Work out the finished part from the listing and answer in its coordinate system (mm). A direction names the side the tool comes from. Coordinates: 2 decimals unless noted, no trailing zeros. Order: outer loops, then holes, each group sorted by start corner. A loop starts at its lowest first (then second) coordinate and runs counter-clockwise, first axis right, second up. Notation, with made-up numbers: M 11.5,-38.75 L 64.5,-38.75 A29 ccw 64.5,-11.75 Z; hole C 32.25,46.25 d2. An arc over 180 degrees is marked long. Use a Markdown table: item, result.
from build123d import *

# Parameters (mm, degrees)
SKETCH1_R                       = 1.15
BOSS_EXTRUDE4_DEPTH             = 3.22
BOSS_EXTRUDE5_DEPTH             = 19
BOSS_EXTRUDE6_DEPTH             = 19
SKETCH3_W                       = 19
SKETCH3_H                       = 8.72
CUT_EXTRUDE1_DEPTH              = 93.159937036
SKETCH2_5_R                     = 6.5
SKETCH2_5_R_2                   = 2.25
SKETCH2_5_W                     = 6.12
SKETCH2_5_H                     = 9.37
BOSS_EXTRUDE9_DEPTH             = 3
BOSS_EXTRUDE9_DEPTH_BACK        = 2
CUT_EXTRUDE8_REACH              = 94.16
SKETCH2_6_W                     = 64
SKETCH2_6_H                     = 14.977988196
CUT_EXTRUDE8_DIRECTION_2_REACH  = 94.16
CUT_EXTRUDE10_REACH             = 94.825
SKETCH4_W                       = 22.69
SKETCH4_H                       = 19
CUT_EXTRUDE10_DIRECTION_2_DEPTH = 3
CUT_EXTRUDE11_REACH             = 93.768
SKETCH5_W                       = 12.894145303
SKETCH5_H                       = 8.72


with BuildPart() as part:
    # Sketch1 → Boss-Extrude4 (new body)
    with BuildSketch(Plane.XY):
        with BuildLine():
            ThreePointArc((2.480923897, -4.488118441), (3.840990258, -3.840990258), (4.488118441, -2.480923897))
            Line((4.488118441, -2.480923897), (2.480923897, -4.488118441))
        make_face()
        with BuildLine():
            Line((2.480923897, -4.488118441), (4.488118441, -2.480923897))
            ThreePointArc((4.488118441, -2.480923897), (4.497027647, -2.365614681), (4.5, -2.25))
            ThreePointArc((4.5, -2.25), (0.579359589, -0.742863438), (2.480923897, -4.488118441))
        make_face()
        with Locations(Location((2.25, -2.25, 0), (0, 0, 180))):
            Circle(SKETCH1_R, mode=Mode.SUBTRACT)
        with BuildLine():
            ThreePointArc((4.5, -47.75), (4.497027647, -47.634385319), (4.488118441, -47.519076103))
            Line((4.488118441, -47.519076103), (2.480923897, -45.511881559))
            ThreePointArc((2.480923897, -45.511881559), (0.579359589, -49.257136562), (4.5, -47.75))
        make_face()
        with Locations(Location((2.25, -47.75, 0), (0, 0, 180))):
            Circle(SKETCH1_R, mode=Mode.SUBTRACT)
        with BuildLine():
            Line((2.480923897, -45.511881559), (4.488118441, -47.519076103))
            ThreePointArc((4.488118441, -47.519076103), (3.840990258, -46.159009742), (2.480923897, -45.511881559))
        make_face()
        with BuildLine():
            Line((67.519076103, -45.511881559), (65.511881559, -47.519076103))
            ThreePointArc((65.511881559, -47.519076103), (67.634385319, -49.997027647), (70, -47.75))
            ThreePointArc((70, -47.75), (69.257136562, -46.079359589), (67.519076103, -45.511881559))
        make_face()
        with Locations(Location((67.75, -47.75, 0), (0, 0, 180))):
            Circle(SKETCH1_R, mode=Mode.SUBTRACT)
        with BuildLine():
            ThreePointArc((67.519076103, -45.511881559), (66.159009742, -46.159009742), (65.511881559, -47.519076103))
            Line((65.511881559, -47.519076103), (67.519076103, -45.511881559))
        make_face()
        with BuildLine():
            ThreePointArc((70, -2.25), (67.634385319, -0.002972353), (65.511881559, -2.480923897))
            Line((65.511881559, -2.480923897), (67.519076103, -4.488118441))
            ThreePointArc((67.519076103, -4.488118441), (69.257136562, -3.920640411), (70, -2.25))
        make_face()
        with Locations(Location((67.75, -2.25, 0), (0, 0, 180))):
            Circle(SKETCH1_R, mode=Mode.SUBTRACT)
        with BuildLine():
            Line((67.519076103, -4.488118441), (65.511881559, -2.480923897))
            ThreePointArc((65.511881559, -2.480923897), (66.159009742, -3.840990258), (67.519076103, -4.488118441))
        make_face()
    extrude(amount=BOSS_EXTRUDE4_DEPTH)

    # Sketch1<6> → Boss-Extrude5 (add)
    with BuildSketch(Plane.XY):
        with BuildLine():
            Line((65.511881559, -47.519076103), (63.030957663, -50))
            ThreePointArc((63.030957663, -50), (71.446745906, -51.446745906), (70, -43.030957663))
            Line((70, -43.030957663), (67.519076103, -45.511881559))
            ThreePointArc((67.519076103, -45.511881559), (69.340990258, -49.340990258), (65.511881559, -47.519076103))
        make_face()
        with BuildLine():
            ThreePointArc((70, -6.969042337), (71.446745906, 1.446745906), (63.030957663, 0))
            Line((63.030957663, 0), (65.511881559, -2.480923897))
            ThreePointArc((65.511881559, -2.480923897), (69.340990258, -0.659009742), (67.519076103, -4.488118441))
            Line((67.519076103, -4.488118441), (70, -6.969042337))
        make_face()
        with BuildLine():
            Line((4.488118441, -2.480923897), (6.969042337, 0))
            ThreePointArc((6.969042337, 0), (-1.446745906, 1.446745906), (0, -6.969042337))
            Line((0, -6.969042337), (2.480923897, -4.488118441))
            ThreePointArc((2.480923897, -4.488118441), (0.659009742, -0.659009742), (4.488118441, -2.480923897))
        make_face()
        with BuildLine():
            ThreePointArc((0, -43.030957663), (-1.446745906, -51.446745906), (6.969042337, -50))
            Line((6.969042337, -50), (4.488118441, -47.519076103))
            ThreePointArc((4.488118441, -47.519076103), (0.659009742, -49.340990258), (2.480923897, -45.511881559))
            Line((2.480923897, -45.511881559), (0, -43.030957663))
        make_face()
    extrude(amount=BOSS_EXTRUDE5_DEPTH)

    # Sketch2 → Boss-Extrude6 (add)
    with BuildSketch(Plane.XY.offset(19)):
        with BuildLine():
            Line((0, -43.030957663), (0, -6.969042337))
            ThreePointArc((0, -6.969042337), (-2.171246093, -5.040061571), (-2.977988196, -2.25))
            Line((-2.977988196, -2.25), (-2.977988196, -47.75))
            ThreePointArc((-2.977988196, -47.75), (-2.171246093, -44.959938429), (0, -43.030957663))
        make_face()
        with BuildLine():
            Line((67.75, 2.977988196), (2.25, 2.977988196))
            ThreePointArc((2.25, 2.977988196), (5.040061571, 2.171246093), (6.969042337, 0))
            Line((6.969042337, 0), (63.030957663, 0))
            ThreePointArc((63.030957663, 0), (64.959938429, 2.171246093), (67.75, 2.977988196))
        make_face()
        with BuildLine():
            Line((2.25, -52.977988196), (67.75, -52.977988196))
            ThreePointArc((67.75, -52.977988196), (64.959938429, -52.171246093), (63.030957663, -50))
            Line((63.030957663, -50), (6.969042337, -50))
            ThreePointArc((6.969042337, -50), (5.040061571, -52.171246093), (2.25, -52.977988196))
        make_face()
        with BuildLine():
            Line((72.977988196, -47.75), (72.977988196, -2.25))
            ThreePointArc((72.977988196, -2.25), (72.171246093, -5.040061571), (70, -6.969042337))
            Line((70, -6.969042337), (70, -43.030957663))
            ThreePointArc((70, -43.030957663), (72.171246093, -44.959938429), (72.977988196, -47.75))
        make_face()
    extrude(amount=-BOSS_EXTRUDE6_DEPTH)

    # Sketch3 → Cut-Extrude1 (cut, through all)
    with BuildSketch(Plane(origin=(0, 0, 0), x_dir=(0, 0, -1), z_dir=(1, 0, 0))):
        with Locations((-9.5, -13.08)):
            Rectangle(SKETCH3_W, SKETCH3_H)
    extrude(amount=-CUT_EXTRUDE1_DEPTH, mode=Mode.SUBTRACT)

    # Sketch2<5> → Boss-Extrude9 (add, two sides)
    with BuildSketch(Plane.XY.offset(19)) as boss_extrude9_sk:
        with BuildLine():
            Line((2.25, -52.977988196), (67.75, -52.977988196))
            ThreePointArc((67.75, -52.977988196), (71.446745906, -51.446745906), (72.977988196, -47.75))
            Line((72.977988196, -47.75), (72.977988196, -2.25))
            ThreePointArc((72.977988196, -2.25), (71.446745906, 1.446745906), (67.75, 2.977988196))
            Line((67.75, 2.977988196), (2.25, 2.977988196))
            ThreePointArc((2.25, 2.977988196), (-1.446745906, 1.446745906), (-2.977988196, -2.25))
            Line((-2.977988196, -2.25), (-2.977988196, -47.75))
            ThreePointArc((-2.977988196, -47.75), (-1.446745906, -51.446745906), (2.25, -52.977988196))
        make_face()
        with BuildLine():
            Line((3, -50), (2.25, -50))
            ThreePointArc((2.25, -50), (0.032403241, -47.369520548), (3, -45.628679656))
            Line((3, -45.628679656), (3, -50))
        make_face(mode=Mode.SUBTRACT)
        with Locations((17.28, -30.89)):
            Circle(SKETCH2_5_R, mode=Mode.SUBTRACT)
        with BuildLine():
            ThreePointArc((67, -45.628679656), (69.967596759, -47.369520548), (67.75, -50))
            Line((67.75, -50), (67, -50))
            Line((67, -50), (67, -45.628679656))
        make_face(mode=Mode.SUBTRACT)
        with Locations(Location((2.25, -2.25, 0), (0, 0, 275.890801568))):
            Circle(SKETCH2_5_R_2, mode=Mode.SUBTRACT)
        with Locations((43.23, -13)):
            Rectangle(SKETCH2_5_W, SKETCH2_5_H, mode=Mode.SUBTRACT)
        with Locations(Location((67.75, -2.25, 0), (0, 0, 185.890801568))):
            Circle(SKETCH2_5_R_2, mode=Mode.SUBTRACT)
    extrude(amount=BOSS_EXTRUDE9_DEPTH)
    extrude(boss_extrude9_sk.sketch, amount=-BOSS_EXTRUDE9_DEPTH_BACK)

    # Sketch2<6> → Cut-Extrude8 (cut, up to next)
    with BuildSketch(Plane.XY.offset(19), mode=Mode.PRIVATE) as cut_extrude8_sk1:
        with Locations((35, -45.488994098)):
            Rectangle(SKETCH2_6_W, SKETCH2_6_H)
    cut_extrude8_tool1 = extrude(cut_extrude8_sk1.sketch, amount=-CUT_EXTRUDE8_REACH, mode=Mode.PRIVATE) & part.part
    add(cut_extrude8_tool1.solids().sort_by_distance((35, -45.488994, 19))[0], mode=Mode.SUBTRACT)

    # Sketch2<6> → Cut-Extrude8 direction 2 (cut, up to next)
    with BuildSketch(Plane.XY.offset(19), mode=Mode.PRIVATE) as cut_extrude8_direction_2_sk1:
        with Locations((35, -45.488994098)):
            Rectangle(SKETCH2_6_W, SKETCH2_6_H)
    cut_extrude8_direction_2_tool1 = extrude(cut_extrude8_direction_2_sk1.sketch, amount=CUT_EXTRUDE8_DIRECTION_2_REACH, mode=Mode.PRIVATE) & part.part
    add(cut_extrude8_direction_2_tool1.solids().sort_by_distance((35, -45.488994, 19))[0], mode=Mode.SUBTRACT)

    # Sketch4 → Cut-Extrude10 (cut, up to next)
    with BuildSketch(Plane.XZ, mode=Mode.PRIVATE) as cut_extrude10_sk1:
        with Locations((54.295, 9.5)):
            Rectangle(SKETCH4_W, SKETCH4_H)
    cut_extrude10_tool1 = extrude(cut_extrude10_sk1.sketch, amount=-CUT_EXTRUDE10_REACH, mode=Mode.PRIVATE) & part.part
    add(cut_extrude10_tool1.solids().sort_by_distance((54.295, 0, 9.5))[0], mode=Mode.SUBTRACT)

    # Sketch4 → Cut-Extrude10 direction 2 (cut)
    with BuildSketch(Plane.XZ):
        with Locations((54.295, 9.5)):
            Rectangle(SKETCH4_W, SKETCH4_H)
    extrude(amount=CUT_EXTRUDE10_DIRECTION_2_DEPTH, mode=Mode.SUBTRACT)

    # Sketch5 → Cut-Extrude11 (cut, up to next)
    with BuildSketch(Plane(origin=(0, 0, 17), x_dir=(-1, 0, 0), z_dir=(0, 0, -1)), mode=Mode.PRIVATE) as cut_extrude11_sk1:
        with Locations((-3.469084455, -13.08)):
            Rectangle(SKETCH5_W, SKETCH5_H)
    cut_extrude11_tool1 = extrude(cut_extrude11_sk1.sketch, amount=-CUT_EXTRUDE11_REACH, mode=Mode.PRIVATE) & part.part
    add(cut_extrude11_tool1.solids().sort_by_distance((3.469084, -13.08, 17))[0], mode=Mode.SUBTRACT)


solid = part.part
(1) A cutting plane is placed at B-B (x = 18). Determine the outline of the cut face in (y, z), then the cut area to 3 significant figures.
Conclusion:
| item | result |
|---|---|
| outline | M -38,17 L -37.35,17 L -37.35,22 L -38,22 Z; M -24.43,17 L 0,17 L 0,0 L 2.98,0 L 2.98,22 L -24.43,22 Z |
| area | 191 mm2 |
(2) Determine the mould class of faces 1 (the flat face through (9.916, -13, 19)), 2 (the cylindrical face through (20.279, -36.657, 19.465)), 3 (the flat face through (3, -42, 19)), 4 (the flat face through (72.978, -25, 11)) for opening direction X: pulls with the +X half, pulls with the -X half, needs draft (parallel to the pull), parting line crosses it, or undercut.
Conclusion:
| item | result |
|---|---|
| face 1 | pulls with the -X half |
| face 2 | undercut |
| face 3 | undercut |
| face 4 | pulls with the +X half |
(3) Which of the six approach directions +Z, -Z, +X, -X, +Y, -Y give full straight-line access (tool end or side, diameter ignored) to faces 5 (the flat face through (-1, -17.44, 16)), 6 (the cylindrical face through (66.344, -4.007, 1.587)), 7 (the flat face through (67, -51, 11)), 8 (the flat face through (1, -47, 3.22)), 9 (the flat face through (54, -3, 18))?
Conclusion:
| item | result |
|---|---|
| face 5 | +Z, -Z, -X |
| face 6 | -Z |
| face 7 | +Z, -Z, -Y |
| face 8 | +Z |
| face 9 | -Z, +Y |
(4) Given P1, Ø1.3, axis at x = 68, y = -1.5, coming from the +Z side; P2, Ø0.9, axis at x = 54.5, y = -1, coming from the -Z side; P3, Ø2.5, axis at y = -12, z = 20, coming from the -X side, each flat-ended and moving along its own axis, determine where each tip first touches the part or whether it passes through.
Conclusion:
| item | result |
|---|---|
| P1 | z = 3.22 |
| P2 | z = 19 |
| P3 | x = 9.92 |
(5) A cutting plane is placed at C-C (z = 2). Give the number of separate pieces and of enclosed holes in the cut face, then the cut area to 3 significant figures.
Conclusion:
| item | result |
|---|---|
| separate pieces | 3 |
| enclosed holes | 2 |
| area | 507 mm2 |
(6) A cutting plane is placed at D-D (y = -30.89). Determine the outline of the cut face in (x, z), then the cut area to 3 significant figures.
Conclusion:
| item | result |
|---|---|
| outline | M -2.98,0 L 0,0 L 0,17 L 10.78,17 L 10.78,22 L -2.98,22 Z; M 23.78,17 L 70,17 L 70,0 L 72.98,0 L 72.98,22 L 23.78,22 Z |
| area | 416 mm2 |
(7) Straight lines are drawn through the part: L1, parallel to X at y = -2.25, z = 17.9; L2, parallel to X at y = -22, z = 12; L3, parallel to Y at x = 2.25, z = 17.8. For each, find the intervals that lie inside material, in ascending order.
Conclusion:
| item | result |
|---|---|
| L1 | -2.98 to 0, 4.5 to 42.95, 70 to 72.98 |
| L2 | -2.98 to 0, 70 to 72.98 |
| L3 | -52.98 to -50, -45.5 to -17.44, -8.72 to -4.5, 0 to 2.98 |
(8) A cutting plane is placed at A-A (y = -41). Determine the outline of the cut face in (x, z), then the cut area to 3 significant figures.
Conclusion:
| item | result |
|---|---|
| outline | M -2.98,0 L 0,0 L 0,17 L 3,17 L 3,22 L -2.98,22 Z; M 67,17 L 70,17 L 70,0 L 72.98,0 L 72.98,22 L 67,22 Z |
| area | 161 mm2 |
